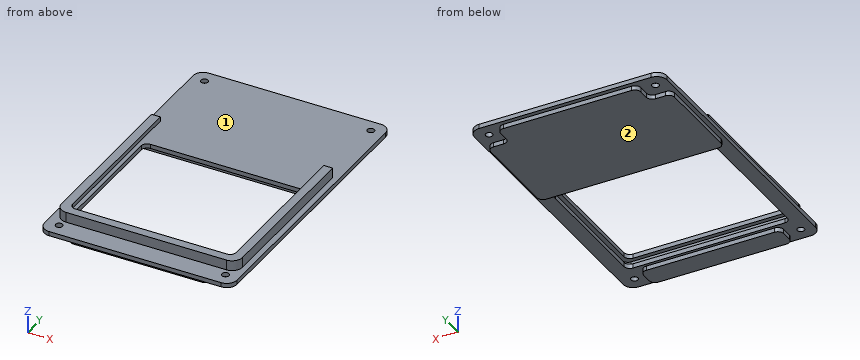
```python
from build123d import *

# Parameters (mm, degrees)
SKETCH_1_W          = 66
SKETCH_1_H          = 100
EXTRUDE_1_DEPTH     = 1.5
FILLET_1_R          = 3.5
SKETCH_2_W          = 56
SKETCH_2_H          = 47
CUT_EXTRUDE_1_DEPTH = 1.5
FILLET_2_R          = 2
EXTRUDE_2_DEPTH     = 2
FILLET_3_R          = 2
EXTRUDE_START       = 1.5
EXTRUDE_3_DEPTH     = 1.5
FILLET_4_R          = 2
FILLET_5_R          = 3.5
SKETCH_5_W          = 48
SKETCH_5_H          = 7.5
EXTRUDE_4_DEPTH     = 1.5
FILLET_6_R          = 2
HOLE_WIZARD_M21_D   = 2.4


with BuildPart() as part:
    # Эскиз1 → Бобышка-Вытянуть1 (new body)
    with BuildSketch(Plane.XY):
        Rectangle(SKETCH_1_W, SKETCH_1_H)
    extrude(amount=EXTRUDE_1_DEPTH)

    # Скругление1
    fillet_1_edges = [part.edges().sort_by_distance(p)[0] for p in [
        (-33, -50, 0.75),
        (-33, 50, 0.75),
        (33, 50, 0.75),
        (33, -50, 0.75),
    ]]
    fillet(fillet_1_edges, radius=FILLET_1_R)

    # Эскиз2 → Вырез-Вытянуть1 (cut)
    with BuildSketch(Plane.XY.offset(1.5)):
        with Locations((0, -16.5)):
            Rectangle(SKETCH_2_W, SKETCH_2_H)
    extrude(amount=-CUT_EXTRUDE_1_DEPTH, mode=Mode.SUBTRACT)

    # Скругление2
    fillet_2_edges = [part.edges().sort_by_distance(p)[0] for p in [
        (28, 7, 0.75),
        (28, -40, 0.75),
        (-28, -40, 0.75),
        (-28, 7, 0.75),
    ]]
    fillet(fillet_2_edges, radius=FILLET_2_R)

    # Эскиз3 → Бобышка-Вытянуть2 (add)
    with BuildSketch(Plane.XY.offset(1.5)):
        Polygon((29.5, -41.5), (-29.5, -41.5), (-29.5, 17), (-31, 17), (-31, -43), (31, -43), (31, 17), (29.5, 17), align=None)
    extrude(amount=EXTRUDE_2_DEPTH)

    # Скругление3
    fillet_3_edges = [part.edges().sort_by_distance(p)[0] for p in [
        (29.5, -41.5, 2.5),
        (-29.5, -41.5, 2.5),
    ]]
    fillet(fillet_3_edges, radius=FILLET_3_R)

    # Эскиз4 → Бобышка-Вытянуть3 (add)
    with BuildSketch(Plane.XY.offset(3.5).offset(EXTRUDE_START)):
        with BuildLine():
            Line((-31, -43), (31, -43))
            Line((31, -43), (31, 17))
            Line((31, 17), (29.5, 17))
            Line((29.5, 17), (29.5, -39.5))
            ThreePointArc((29.5, -39.5), (28.914213562, -40.914213562), (27.5, -41.5))
            Line((27.5, -41.5), (-27.5, -41.5))
            ThreePointArc((-27.5, -41.5), (-28.914213562, -40.914213562), (-29.5, -39.5))
            Line((-29.5, -39.5), (-29.5, 17))
            Line((-29.5, 17), (-31, 17))
            Line((-31, 17), (-31, -43))
        make_face()
        with BuildLine():
            Line((-28, 17), (-29.5, 17))
            Line((-29.5, 17), (-29.5, -39.5))
            ThreePointArc((-29.5, -39.5), (-28.914213562, -40.914213562), (-27.5, -41.5))
            Line((-27.5, -41.5), (27.5, -41.5))
            ThreePointArc((27.5, -41.5), (28.914213562, -40.914213562), (29.5, -39.5))
            Line((29.5, -39.5), (29.5, 17))
            Line((29.5, 17), (28, 17))
            Line((28, 17), (28, -40))
            Line((28, -40), (-28, -40))
            Line((-28, -40), (-28, 17))
        make_face()
    extrude(amount=-EXTRUDE_3_DEPTH)

    # Скругление4
    fillet_4_edges = [part.edges().sort_by_distance(p)[0] for p in [
        (28, -40, 4.25),
        (-28, -40, 4.25),
    ]]
    fillet(fillet_4_edges, radius=FILLET_4_R)

    # Скругление5
    fillet_5_edges = [part.edges().sort_by_distance(p)[0] for p in [
        (31, -43, 3.25),
        (-31, -43, 3.25),
    ]]
    fillet(fillet_5_edges, radius=FILLET_5_R)

    # Эскиз5 → Бобышка-Вытянуть4 (add)
    with BuildSketch(Plane(origin=(0, 0, 0), x_dir=(-1, 0, 0), z_dir=(0, 0, -1))):
        Polygon((24, 48.5), (-24, 48.5), (-24, 41), (-31.5, 41), (-31.5, 8), (31.5, 8), (31.5, 41), (24, 41), align=None)
        with Locations((0, -44.75)):
            Rectangle(SKETCH_5_W, SKETCH_5_H)
    extrude(amount=EXTRUDE_4_DEPTH)

    # Скругление6
    fillet_6_edges = [part.edges().sort_by_distance(p)[0] for p in [
        (-24, 48.5, -0.75),
        (24, 48.5, -0.75),
        (24, 41, -0.75),
        (31.5, 41, -0.75),
        (31.5, 8, -0.75),
        (-31.5, 8, -0.75),
        (-31.5, 41, -0.75),
        (-24, 41, -0.75),
        (-24, -48.5, -0.75),
        (-24, -41, -0.75),
        (24, -41, -0.75),
        (24, -48.5, -0.75),
    ]]
    fillet(fillet_6_edges, radius=FILLET_6_R)

    # Отверстие с зазором M21 (through all)
    with Locations(Plane.XY.offset(1.5)):
        with Locations((-28.5, 45.5), (28.5, 45.5), (28.5, -45.5), (-28.5, -45.5)):
            Hole(HOLE_WIZARD_M21_D / 2)


solid = part.part
```
Verification items for the finished model (mm, model axes). Face numbers are marked on the shaded views. Coordinates: 2 decimals unless noted, no trailing zeros. Loops run counter-clockwise (first coordinate to the right, second up) from the corner with the lowest first, then second, coordinate; pieces in that order, holes last. Notation, with made-up numbers: (-11, 10.5) -> (-1, 10.5) arc R23 ccw to (-1, 39.5) -> close; hole circle Ø4 at (-7, 14). An arc over 180 degrees is marked (long way). Put each result on its own line as item: value.
1. Mould release check, pull along X, two halves, no side actions. Record for the marked faces 1 and 2: pulls with the +X half, pulls with the -X half, needs draft (parallel to the pull), parting line crosses it, or undercut.
Result set:
face 1: undercut
face 2: needs draft
2. Section check A-A, the plane y = -30. Record the boundary of the cut face in (x, z), then the cut area to 3 significant figures.
Result set:
outline: (-33, 0) -> (-28, 0) -> (-28, 1.5) -> (-29.5, 1.5) -> (-29.5, 3.5) -> (-28, 3.5) -> (-28, 5) -> (-31, 5) -> (-31, 1.5) -> (-33, 1.5) -> close; (28, 0) -> (33, 0) -> (33, 1.5) -> (31, 1.5) -> (31, 5) -> (28, 5) -> (28, 3.5) -> (29.5, 3.5) -> (29.5, 1.5) -> (28, 1.5) -> close
area: 30.0 mm^2
3. Section check C-C, the plane x = -14. Record the boundary of the cut face in (y, z), then the cut area to 3 significant figures.
Result set:
outline: (-50, 0) -> (-48.5, 0) -> (-48.5, -1.5) -> (-41, -1.5) -> (-41, 0) -> (-40, 0) -> (-40, 1.5) -> (-41.5, 1.5) -> (-41.5, 3.5) -> (-40, 3.5) -> (-40, 5) -> (-43, 5) -> (-43, 1.5) -> (-50, 1.5) -> close; (7, 0) -> (8, 0) -> (8, -1.5) -> (48.5, -1.5) -> (48.5, 0) -> (50, 0) -> (50, 1.5) -> (7, 1.5) -> close
area: 159 mm^2
4. Thickness scan on line 1 (Y direction, x = 28.5, z = 1.1); line 2 (X direction, y = 8.5, z = 4.5); line 3 (X direction, y = -39.5, z = 1). Record the ranges inside material, lowest first.
Result set:
line 1: y = -50 to -46.7, -44.3 to 44.3, 46.7 to 50
line 2: x = -31 to -28, 28 to 31
line 3: x = -33 to -27.32, 27.32 to 33
5. Section check B-B, the plane y = 45.5. Record the boundary of the cut face in (x, z), then the cut area to 3 significant figures.
Result set:
outline: (-33, 0) -> (-29.7, 0) -> (-29.7, 1.5) -> (-33, 1.5) -> close; (-27.3, 0) -> (-24, 0) -> (-24, -1.5) -> (24, -1.5) -> (24, 0) -> (27.3, 0) -> (27.3, 1.5) -> (-27.3, 1.5) -> close; (29.7, 0) -> (33, 0) -> (33, 1.5) -> (29.7, 1.5) -> close
area: 164 mm^2
6. Section check D-D, the plane y = 28. Record the boundary of the cut face in (x, z), then the cut area to 4 significant figures.
Result set:
outline: (-33, 0) -> (-31.5, 0) -> (-31.5, -1.5) -> (31.5, -1.5) -> (31.5, 0) -> (33, 0) -> (33, 1.5) -> (-33, 1.5) -> close
area: 193.5 mm^2
7. Gauge pin test, flat ends, axial feed: P1, Ø1.5, axis at y = 1.5, z = 4, coming from the +X side; P2, Ø1.2, axis at y = -45.5, z = -1, coming from the -X side; P3, Ø1.6, axis at y = -45.5, z = -1, coming from the +X side; P4, Ø1.4, axis at x = -28.5, y = -45.5, coming from the -Z side. Record the tip position at first contact, or that the pin passes through.
Result set:
P1: stops at x = 31
P2: stops at x = -24
P3: stops at x = 24
P4: passes through
